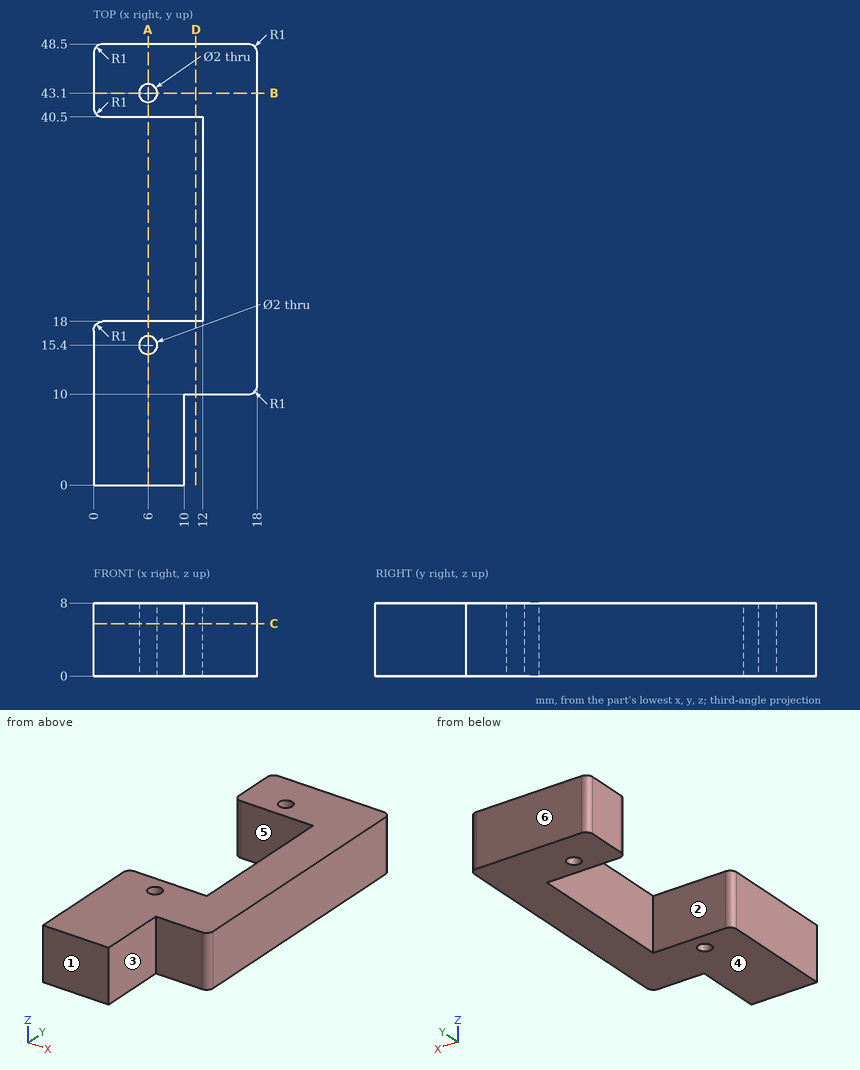
Job drawing, mm, ordinate dimensions from the low corner. One solid piece. A direction names the side the tool comes from. Coordinates: 2 decimals unless noted, no trailing zeros. Order: outer loops, then holes, each group sorted by start corner. A loop starts at its lowest first (then second) coordinate and runs counter-clockwise, first axis right, second up. Notation, with made-up numbers: (47.5, -31.75) - (98.5, -31.75) arc R13 ccw to (98.5, -23.75) - close; hole circle Ø7 at (-19.5, 18). An arc over 180 degrees is marked (long way). Use CSV: the item, a comma, the result in double quotes.
Item 1: Saw through at C-C on z = 5.75. Give the cut face in (x, y), and give its area (3 significant figures).
Solved:
outline,"(0, 0) - (10, 0) - (10, 10) - (17, 10) arc R1 ccw to (18, 11) - (18, 47.5) arc R1 ccw to (17, 48.5) - (1, 48.5) arc R1 ccw to (0, 47.5) - (0, 41.5) arc R1 ccw to (1, 40.5) - (12, 40.5) - (12, 18) - (1, 18) arc R1 ccw to (0, 17) - close; hole circle Ø2 at (6, 15.4); hole circle Ø2 at (6, 43.1)"
area,"516 mm²"
Item 2: Mould opens along Y. For the marked faces 4, 5 and 6 say: +Y half, -Y half, draft (parallel to the pull), parting line (faces both ways), or undercut.
Solved:
face 4,"draft"
face 5,"undercut"
face 6,"+Y half"
Item 3: Saw through at A-A on x = 6. Give the cut face in (y, z).
Solved:
outline,"(0, 0) - (14.4, 0) - (14.4, 8) - (0, 8) - close; (16.4, 0) - (18, 0) - (18, 8) - (16.4, 8) - close; (40.5, 0) - (42.1, 0) - (42.1, 8) - (40.5, 8) - close; (44.1, 0) - (48.5, 0) - (48.5, 8) - (44.1, 8) - close"
Item 4: Drop a flat-ended pin along its axis: P1, Ø2, axis at x = 12.5, z = 5, coming from the -Y side. Give the stop position or say it passes through.
Solved:
P1,"stops at y = 10"
Item 5: Probe probe 1 along Y at (x, z) = (6, 3.25); probe 2 along Y at (x, z) = (9.5, 2.25); probe 3 along X at (y, z) = (36, 4.75). List the from-to ranges inside material, lowest first.
Solved:
probe 1,"y = 0 to 14.4, 16.4 to 18, 40.5 to 42.1, 44.1 to 48.5"
probe 2,"y = 0 to 18, 40.5 to 48.5"
probe 3,"x = 12 to 18"
Item 6: 3-axis set-ups, long thin cutter, end or side, ignore diameter. For the marked faces 1, 2 and 3: which of +Z, -Z, +X, -X, +Y, -Y reach the whole face in a straight line?
Solved:
face 1,"+Z, -Z, +X, -X, -Y"
face 2,"+Z, -Z, -X"
face 3,"+Z, -Z, +X, -Y"
Item 7: Saw through at B-B on y = 43.1. Give the cut face in (x, z), and give its area (3 significant figures).
Solved:
outline,"(0, 0) - (5, 0) - (5, 8) - (0, 8) - close; (7, 0) - (18, 0) - (18, 8) - (7, 8) - close"
area,"128 mm²"
Item 8: Saw through at D-D on x = 11.25. Give the cut face in (y, z).
Solved:
outline,"(10, 0) - (18, 0) - (18, 8) - (10, 8) - close; (40.5, 0) - (48.5, 0) - (48.5, 8) - (40.5, 8) - close"
